Geometry check sheet. Reference: the model listing, model coordinates, mm. Face numbers are marked on the shaded views. A direction names the side the tool comes from. Give positions to 0.01 mm unless a question says otherwise; leave off trailing zeros. Write each loop counter-clockwise with the first axis right and the second up, starting at its lowest first coordinate (ties: lowest second). Pieces come first, ordered by that corner, then holes. Notation, with made-up numbers: M -8,25 L 31,25 A13 cw 31,37 Z; hole C -15,69 d6. An arc over 180 degrees is marked long. One line per item, written item: value. Start each with the question number.
1. Cross-section at A-A on y = 8. Record the cut outline in (x, z), then the cut area to 3 significant figures.
2. Scan lines: line 1 (X direction, y = 23, z = 31.5); line 2 (Y direction, x = -43.5, z = 3.5); line 3 (Z direction, x = -15, y = 9.5). Record each from-to range of solid material in increasing order.
3. Tool access check on the marked faces 4, 5, 6, 7 and 8. Record the directions out of +Z, -Z, +X, -X, +Y, -Y that give a thin tool (end or side, any length) a straight path to the whole face; none if there is none.
4. Release check for a two-part mould opening along X. For the marked faces 1, 2 and 3 record: pulls with the +X half, pulls with the -X half, needs draft (parallel to the pull), parting line crosses it, or undercut.
5. Cross-section at B-B on z = 7.5. Record the cut outline in (x, y), then the cut area to 3 significant figures.
6. Gauge pin test, flat ends, axial feed: pin 1 (2 mm diameter, centred on y = 24, z = 15.5, fed in from +X); pin 2 (9 mm diameter, centred on x = -43.5, y = 24, fed in from +Z); pin 3 (4 mm diameter, centred on x = -29.5, z = 29.5, fed in from +Y); pin 4 (0.6 mm diameter, centred on y = 30.5, z = 24, fed in from -X). Record the tip position at first contact, or that the pin passes through.
7. Cross-section at D-D on x = -33. Record the cut outline in (y, z).
8. Cross-section at C-C on x = -51. Record the cut outline in (y, z), then the cut area to 3 significant figures.
from build123d import *

# Parameters (mm, degrees)
CROQUIS1_W              = 62.2
CROQUIS1_H              = 44.7
SALIENTE_EXTRUIR1_DEPTH = 24.5
CROQUIS2_W              = 32
CROQUIS2_H              = 28.7
SALIENTE_EXTRUIR2_DEPTH = 8.5
CROQUIS3_W              = 18
CROQUIS3_H              = 18
CORTAR_EXTRUIR1_DEPTH   = 0.5
CROQUIS4_W              = 13
CROQUIS4_H              = 13
SALIENTE_EXTRUIR3_DEPTH = 1
REDONDEO2_R             = 0.5
REDONDEO3_R             = 1
REDONDEO1_R             = 4


with BuildPart() as part:
    # Croquis1 → Saliente-Extruir1 (new body)
    with BuildSketch(Plane.XY):
        with Locations((-31.1, 22.35)):
            Rectangle(CROQUIS1_W, CROQUIS1_H)
    extrude(amount=SALIENTE_EXTRUIR1_DEPTH)

    # Croquis2 → Saliente-Extruir2 (add)
    with BuildSketch(Plane.XY.offset(24.5)):
        with Locations((-16, 30.35)):
            Rectangle(CROQUIS2_W, CROQUIS2_H)
    extrude(amount=SALIENTE_EXTRUIR2_DEPTH)

    # Croquis3 → Cortar-Extruir1 (cut)
    with BuildSketch(Plane.XY.offset(24.5)):
        with Locations((-46, 27)):
            Rectangle(CROQUIS3_W, CROQUIS3_H)
    extrude(amount=-CORTAR_EXTRUIR1_DEPTH, mode=Mode.SUBTRACT)

    # Croquis4 → Saliente-Extruir3 (add)
    with BuildSketch(Plane(origin=(0, 44.7, 0), x_dir=(1, 0, 0), z_dir=(0, 1, 0))):
        with Locations((-46.7, -11.5)):
            Rectangle(CROQUIS4_W, CROQUIS4_H)
    extrude(amount=SALIENTE_EXTRUIR3_DEPTH)

    # Redondeo2
    redondeo2_edges = [part.edges().sort_by_distance(p)[0] for p in [
        (-55, 18, 24.25),
        (-55, 36, 24.25),
        (-37, 36, 24.25),
        (-37, 18, 24.25),
        (-40.2, 44.7, 11.5),
        (-40.2, 45.2, 18),
        (-46.7, 44.7, 5),
        (-40.2, 45.2, 5),
        (-53.2, 44.7, 11.5),
        (-53.2, 45.2, 5),
        (-46.7, 44.7, 18),
        (-53.2, 45.2, 18),
    ]]
    fillet(redondeo2_edges, radius=REDONDEO2_R)

    # Redondeo3
    redondeo3_edges = [part.edges().sort_by_distance(p)[0] for p in [
        (-31.1, 0, 0),
        (-62.2, 22.35, 0),
        (-31.1, 44.7, 0),
        (0, 22.35, 0),
    ]]
    fillet(redondeo3_edges, radius=REDONDEO3_R)

    # Redondeo1
    # the kernel refuses this fillet: 4 mm, written as the material it takes off along each edge
    with BuildSketch(Plane(origin=(-4, 40.7, 0), x_dir=(0, 1, 0), z_dir=(-1, 0, 0))) as redondeo1_piece_1:
        with BuildLine():
            CenterArc((3, -1), 1, 0, 90)
            Line((4, -1), (4, 0))
            Line((4, 0), (3, 0))
        make_face()
    revolve(axis=Axis((-4, 40.7, 0), (0, 0, -1)), revolution_arc=90, mode=Mode.SUBTRACT)
    with BuildSketch(Plane(origin=(-4, 4, 0), x_dir=(1, 0, 0), z_dir=(0, 1, 0))) as redondeo1_piece_2:
        with BuildLine():
            CenterArc((3, -1), 1, 0, 90)
            Line((4, -1), (4, 0))
            Line((4, 0), (3, 0))
        make_face()
    revolve(axis=Axis((-4, 4, 0), (0, 0, -1)), revolution_arc=90, mode=Mode.SUBTRACT)
    with BuildSketch(Plane(origin=(-58.2, 40.7, 0), x_dir=(-1, 0, 0), z_dir=(0, -1, 0))) as redondeo1_piece_3:
        with BuildLine():
            CenterArc((3, -1), 1, 0, 90)
            Line((4, -1), (4, 0))
            Line((4, 0), (3, 0))
        make_face()
    revolve(axis=Axis((-58.2, 40.7, 0), (0, 0, -1)), revolution_arc=90, mode=Mode.SUBTRACT)
    with BuildSketch(Plane(origin=(-58.2, 4, 0), x_dir=(0, -1, 0), z_dir=(1, 0, 0))) as redondeo1_piece_4:
        with BuildLine():
            CenterArc((3, -1), 1, 0, 90)
            Line((4, -1), (4, 0))
            Line((4, 0), (3, 0))
        make_face()
    revolve(axis=Axis((-58.2, 4, 0), (0, 0, -1)), revolution_arc=90, mode=Mode.SUBTRACT)
    with BuildSketch(Plane(origin=(-58.2, 4, 20.5), x_dir=(0, 0, 1), z_dir=(0, -1, 0))) as redondeo1_piece_5_section:
        Polygon((0, 0), (REDONDEO1_R, 0), (REDONDEO1_R, REDONDEO1_R), (0, REDONDEO1_R), align=None)
    redondeo1_piece_5 = extrude(amount=REDONDEO1_R, mode=Mode.PRIVATE)
    redondeo1_piece_5 = redondeo1_piece_5 - Plane(origin=(-58.2, 4, 20.5), x_dir=(0.7071067811865475, 0, -0.7071067811865475), z_dir=(0, -1, 0)) * Sphere(REDONDEO1_R, mode=Mode.PRIVATE)
    add(redondeo1_piece_5, mode=Mode.SUBTRACT)
    with BuildSketch(Plane(origin=(-58.2, 40.7, 20.5), x_dir=(0, 0, 1), z_dir=(0, 1, 0))) as redondeo1_piece_6_section:
        Polygon((0, 0), (REDONDEO1_R, 0), (REDONDEO1_R, -REDONDEO1_R), (0, -REDONDEO1_R), align=None)
    redondeo1_piece_6 = extrude(amount=REDONDEO1_R, mode=Mode.PRIVATE)
    redondeo1_piece_6 = redondeo1_piece_6 - Plane(origin=(-58.2, 40.7, 20.5), x_dir=(0.7071067811865475, 0, -0.7071067811865475), z_dir=(0, 1, 0)) * Sphere(REDONDEO1_R, mode=Mode.PRIVATE)
    add(redondeo1_piece_6, mode=Mode.SUBTRACT)
    with BuildSketch(Plane(origin=(-4, 4, 20.5), x_dir=(0, -1, 0), z_dir=(1, 0, 0))) as redondeo1_piece_7_section:
        Polygon((0, 0), (REDONDEO1_R, 0), (REDONDEO1_R, -REDONDEO1_R), (0, -REDONDEO1_R), align=None)
    redondeo1_piece_7 = extrude(amount=REDONDEO1_R, mode=Mode.PRIVATE)
    redondeo1_piece_7 = redondeo1_piece_7 - Plane(origin=(-4, 4, 20.5), x_dir=(0, 0.7071067811865475, -0.7071067811865475), z_dir=(1, 0, 0)) * Sphere(REDONDEO1_R, mode=Mode.PRIVATE)
    add(redondeo1_piece_7, mode=Mode.SUBTRACT)
    with BuildSketch(Plane(origin=(-62.2, 4, 24.5), x_dir=(1, 0, 0), z_dir=(0, 1, 0))) as redondeo1_piece_8:
        with BuildLine():
            CenterArc((REDONDEO1_R, REDONDEO1_R), REDONDEO1_R, 180, 90)
            Line((0, REDONDEO1_R), (0, 0))
            Line((0, 0), (REDONDEO1_R, 0))
        make_face()
    extrude(amount=36.7, mode=Mode.SUBTRACT)
    with BuildSketch(Plane(origin=(-4, 0, 24.5), x_dir=(0, 0, -1), z_dir=(-1, 0, 0))) as redondeo1_piece_9:
        with BuildLine():
            CenterArc((REDONDEO1_R, -REDONDEO1_R), REDONDEO1_R, 90, 90)
            Line((0, -REDONDEO1_R), (0, 0))
            Line((0, 0), (REDONDEO1_R, 0))
        make_face()
    extrude(amount=54.2, mode=Mode.SUBTRACT)
    with BuildSketch(Plane(origin=(-58.2, 44.7, 24.5), x_dir=(0, 0, -1), z_dir=(1, 0, 0))) as redondeo1_piece_10:
        with BuildLine():
            CenterArc((REDONDEO1_R, -REDONDEO1_R), REDONDEO1_R, 90, 90)
            Line((0, -REDONDEO1_R), (0, 0))
            Line((0, 0), (REDONDEO1_R, 0))
        make_face()
    extrude(amount=26.2, mode=Mode.SUBTRACT)
    with BuildSketch(Plane(origin=(0, 16, 24.5), x_dir=(0, 1, 0), z_dir=(0, 0, 1)), Plane(origin=(-32, 16, 24.5), x_dir=(1, 0, 0), z_dir=(0, 0, 1))) as redondeo1_piece_11:
        with BuildLine():
            CenterArc((REDONDEO1_R, REDONDEO1_R), REDONDEO1_R, 180, 90)
            Line((0, REDONDEO1_R), (0, 0))
            Line((0, 0), (REDONDEO1_R, 0))
        make_face()
    extrude(amount=18.5, mode=Mode.SUBTRACT)
    with BuildSketch(Plane(origin=(-32, 44.7, 24.5), x_dir=(1, 0, 0), z_dir=(0, 0, 1))) as redondeo1_piece_12:
        with BuildLine():
            CenterArc((REDONDEO1_R, -REDONDEO1_R), REDONDEO1_R, 90, 90)
            Line((0, -REDONDEO1_R), (0, 0))
            Line((0, 0), (REDONDEO1_R, 0))
        make_face()
    extrude(amount=18.5, mode=Mode.SUBTRACT)
    with BuildSketch(Plane(origin=(0, 16, 24.5), x_dir=(0, 0, -1), z_dir=(0, -1, 0))) as redondeo1_piece_13:
        with BuildLine():
            CenterArc((REDONDEO1_R, -REDONDEO1_R), REDONDEO1_R, 90, 90)
            Line((0, -REDONDEO1_R), (0, 0))
            Line((0, 0), (REDONDEO1_R, 0))
        make_face()
    extrude(amount=12, mode=Mode.SUBTRACT)
    with BuildSketch(Plane(origin=(0, 0, 0), x_dir=(0, 1, 0), z_dir=(0, 0, 1)), Plane(origin=(-62.2, 0, 0), x_dir=(1, 0, 0), z_dir=(0, 0, 1))) as redondeo1_piece_14:
        with BuildLine():
            CenterArc((REDONDEO1_R, REDONDEO1_R), REDONDEO1_R, 180, 90)
            Line((0, REDONDEO1_R), (0, 0))
            Line((0, 0), (REDONDEO1_R, 0))
        make_face()
    extrude(amount=20.5, mode=Mode.SUBTRACT)
    with BuildSketch(Plane(origin=(-62.2, 44.7, 0), x_dir=(1, 0, 0), z_dir=(0, 0, 1))) as redondeo1_piece_15:
        with BuildLine():
            CenterArc((REDONDEO1_R, -REDONDEO1_R), REDONDEO1_R, 90, 90)
            Line((0, -REDONDEO1_R), (0, 0))
            Line((0, 0), (REDONDEO1_R, 0))
        make_face()
    extrude(amount=20.5, mode=Mode.SUBTRACT)
    with BuildSketch(Plane(origin=(0, 44.7, 0), x_dir=(0, -1, 0), z_dir=(0, 0, 1))) as redondeo1_piece_16:
        with BuildLine():
            CenterArc((REDONDEO1_R, -REDONDEO1_R), REDONDEO1_R, 90, 90)
            Line((0, -REDONDEO1_R), (0, 0))
            Line((0, 0), (REDONDEO1_R, 0))
        make_face()
    extrude(amount=43, mode=Mode.SUBTRACT)
    with BuildSketch(Plane(origin=(-58.2, 44.7, 24.5), x_dir=(0, 0, -1), z_dir=(1, 0, 0))) as redondeo1_piece_17a_section:
        with BuildLine():
            CenterArc((REDONDEO1_R, -REDONDEO1_R), REDONDEO1_R, 90, 90)
            Line((0, -REDONDEO1_R), (0, 0))
            Line((0, 0), (REDONDEO1_R, 0))
        make_face()
    redondeo1_piece_17a = extrude(amount=36.2, mode=Mode.PRIVATE)
    redondeo1_piece_17a = split(redondeo1_piece_17a, bisect_by=Plane(origin=(-32, 43.794419543, 23.594419543), z_dir=(1, 0, 0)), keep=Keep.TOP, mode=Mode.PRIVATE)
    with BuildSketch(Plane(origin=(-32, 44.7, 14.5), x_dir=(1, 0, 0), z_dir=(0, 0, 1))) as redondeo1_piece_17b_section:
        with BuildLine():
            CenterArc((REDONDEO1_R, -REDONDEO1_R), REDONDEO1_R, 90, 90)
            Line((0, -REDONDEO1_R), (0, 0))
            Line((0, 0), (REDONDEO1_R, 0))
        make_face()
    redondeo1_piece_17b = extrude(amount=28.5, mode=Mode.PRIVATE)
    redondeo1_piece_17b = split(redondeo1_piece_17b, bisect_by=Plane(origin=(-31.094419543, 43.794419543, 24.5), z_dir=(0, 0, -1)), keep=Keep.TOP, mode=Mode.PRIVATE)
    redondeo1_piece_17 = redondeo1_piece_17a & redondeo1_piece_17b
    add(redondeo1_piece_17, mode=Mode.SUBTRACT)
    with BuildSketch(Plane(origin=(0, 16, 14.5), x_dir=(0, 1, 0), z_dir=(0, 0, 1))) as redondeo1_piece_18a_section:
        with BuildLine():
            CenterArc((REDONDEO1_R, REDONDEO1_R), REDONDEO1_R, 180, 90)
            Line((0, REDONDEO1_R), (0, 0))
            Line((0, 0), (REDONDEO1_R, 0))
        make_face()
    redondeo1_piece_18a = extrude(amount=28.5, mode=Mode.PRIVATE)
    redondeo1_piece_18a = split(redondeo1_piece_18a, bisect_by=Plane(origin=(-0.905580457, 16.905580457, 24.5), z_dir=(0, 0, -1)), keep=Keep.TOP, mode=Mode.PRIVATE)
    with BuildSketch(Plane(origin=(0, 26, 24.5), x_dir=(0, 0, -1), z_dir=(0, -1, 0))) as redondeo1_piece_18b_section:
        with BuildLine():
            CenterArc((REDONDEO1_R, -REDONDEO1_R), REDONDEO1_R, 90, 90)
            Line((0, -REDONDEO1_R), (0, 0))
            Line((0, 0), (REDONDEO1_R, 0))
        make_face()
    redondeo1_piece_18b = extrude(amount=22, mode=Mode.PRIVATE)
    redondeo1_piece_18b = split(redondeo1_piece_18b, bisect_by=Plane(origin=(-0.905580457, 16, 23.594419543), z_dir=(0, 1, 0)), keep=Keep.TOP, mode=Mode.PRIVATE)
    redondeo1_piece_18 = redondeo1_piece_18a & redondeo1_piece_18b
    add(redondeo1_piece_18, mode=Mode.SUBTRACT)


solid = part.part
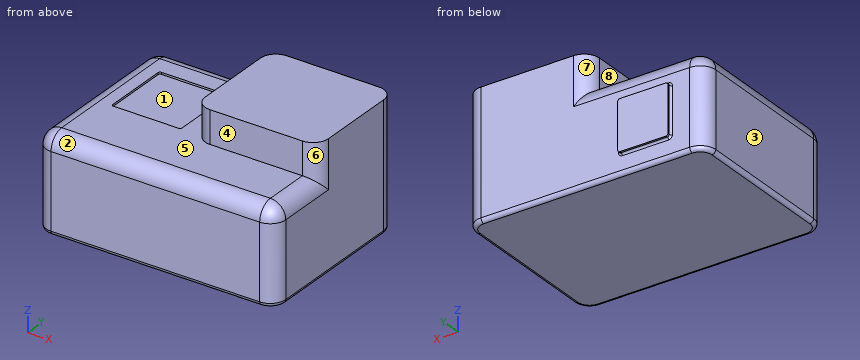
Report:
1. outline: M -62.2,1 A1 ccw -61.2,0 L -1,0 A1 ccw 0,1 L 0,20.5 A4 ccw -4,24.5 L -58.2,24.5 A4 ccw -62.2,20.5 Z
1. area: 1,520 mm^2
2. line 1: x = -32 to 0
2. line 2: y = 0 to 44.7
2. line 3: z = 0 to 24.5
3. face 4: +Z, +X, -X, -Y
3. face 5: +Z, -X, -Y
3. face 6: +Z, +X, -Y
3. face 7: +Z, -X, +Y
3. face 8: +Z, -X, +Y, -Y
4. face 1: undercut
4. face 2: needs draft
4. face 3: pulls with the -X half
5. outline: M -62.2,4 A4 ccw -58.2,0 L -4,0 A4 ccw 0,4 L 0,40.7 A4 ccw -4,44.7 L -39.7,44.7 A0.5 cw -40.2,45.2 L -40.2,45.7 L -53.2,45.7 L -53.2,45.2 A0.5 cw -53.7,44.7 L -58.2,44.7 A4 ccw -62.2,40.7 Z
5. area: 2,780 mm^2
6. pin 1: stops at x = 0
6. pin 2: stops at z = 24
6. pin 3: stops at y = 44.7
6. pin 4: stops at x = -60.6
7. outline: M 0,1 A1 ccw 1,0 L 43.7,0 A1 ccw 44.7,1 L 44.7,20.5 A4 ccw 40.7,24.5 L 4,24.5 A4 ccw 0,20.5 Z
8. outline: M 0,1 A1 ccw 1,0 L 43.7,0 A1 ccw 44.7,1 L 44.7,4.5 A0.5 cw 45.2,5 L 45.7,5 L 45.7,18 L 45.2,18 A0.5 cw 44.7,18.5 L 44.7,20.5 A4 ccw 40.7,24.5 L 36,24.5 L 36,24 L 18,24 L 18,24.5 L 4,24.5 A4 ccw 0,20.5 Z
8. area: 1,090 mm^2
